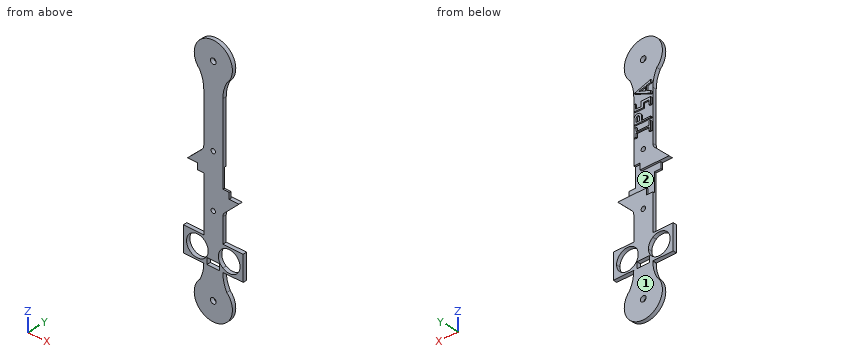
from build123d import *
from build123d.topology import SkipClean

# Parameters (mm, degrees)
SKETCH1_R            = 2
SKETCH1_R_2          = 1.5
BOSS_EXTRUDE2_DEPTH  = 3
SKETCH3_W            = 15.09800494
SKETCH3_H            = 15
CUT_EXTRUDE9_DEPTH   = 1.5
BOSS_EXTRUDE7_DEPTH  = 1.5
BOSS_EXTRUDE9_DEPTH  = 3
SKETCH11_W           = 5
SKETCH11_H           = 5
CUT_EXTRUDE16_DEPTH  = 1.5
SKETCH12_W           = 5
SKETCH12_H           = 5
BOSS_EXTRUDE16_DEPTH = 1.5
BOSS_EXTRUDE17_START = -3
SKETCH15_R           = 1.5
BOSS_EXTRUDE17_DEPTH = 3
SKETCH16_R           = 1.5
CUT_EXTRUDE17_DEPTH  = 103.05738215
BOSS_EXTRUDE23_DEPTH = 1
BOSS_EXTRUDE27_DEPTH = 3
SKETCH27_W           = 5
SKETCH27_H           = 5
CUT_EXTRUDE20_DEPTH  = 3
SKETCH28_R           = 2.25
CUT_EXTRUDE22_DEPTH  = 103.779175528
SKETCH29_R           = 1.75
CUT_EXTRUDE23_DEPTH  = 10


with BuildPart() as part:
    # Sketch1 → Boss-Extrude2 (new body)
    with BuildSketch(Plane(origin=(0, 0, 0), x_dir=(1, 0, 0), z_dir=(0, 1, 0))):
        with BuildLine():
            Line((-7.45099753, -61.780902979), (-7.45099753, 61.780902979))
            ThreePointArc((-7.45099753, 61.780902979), (-8.239083338, 68.275631842), (-10.557599248, 74.393398282))
            ThreePointArc((-10.557599248, 74.393398282), (0.04900247, 100), (10.655604188, 74.393398282))
            ThreePointArc((10.655604188, 74.393398282), (8.337088278, 68.275631842), (7.54900247, 61.780902979))
            Line((7.54900247, 61.780902979), (7.54900247, -61.780902979))
            ThreePointArc((7.54900247, -61.780902979), (8.337088278, -68.275631842), (10.655604188, -74.393398282))
            ThreePointArc((10.655604188, -74.393398282), (0.04900247, -100), (-10.557599248, -74.393398282))
            ThreePointArc((-10.557599248, -74.393398282), (-8.239083338, -68.275631842), (-7.45099753, -61.780902979))
        make_face()
        with Locations(Location((0.04900247, 85, 0), (0, 0, 270))):
            Circle(SKETCH1_R, mode=Mode.SUBTRACT)
        with Locations(Location((0, 20, 0), (0, 0, 270))):
            Circle(SKETCH1_R_2, mode=Mode.SUBTRACT)
        with Locations(Location((0.04900247, -85, 0), (0, 0, 90))):
            Circle(SKETCH1_R, mode=Mode.SUBTRACT)
        with Locations(Location((0, -20, 0), (0, 0, 90))):
            Circle(SKETCH1_R_2, mode=Mode.SUBTRACT)
    extrude(amount=BOSS_EXTRUDE2_DEPTH)

    # Sketch3 → Cut-Extrude9 (cut)
    with BuildSketch(Plane(origin=(0, 3, 0), x_dir=(1, 0, 0), z_dir=(0, 1, 0))):
        Rectangle(SKETCH3_W, SKETCH3_H)
    extrude(amount=-CUT_EXTRUDE9_DEPTH, mode=Mode.SUBTRACT)

    # Sketch4 → Boss-Extrude7 (add, symmetric)
    with BuildSketch(Plane(origin=(0, 1.5, 0), x_dir=(1, 0, 0), z_dir=(0, 1, 0))):
        Polygon((-7.380219176, -20), (-20.167033775, -7.5), (-7.45099753, -7.5), align=None)
        Polygon((7.54900247, 20), (20.167033775, 7.5), (7.54900247, 7.5), align=None)
    extrude(amount=BOSS_EXTRUDE7_DEPTH, both=True)

    # Sketch7 → Boss-Extrude9 (add)
    with BuildSketch(Plane(origin=(0, 3, 0), x_dir=(1, 0, 0), z_dir=(0, 1, 0))):
        with BuildLine():
            Line((-7.45099753, -19.930809239), (-8.881159755, -18.532726263))
            ThreePointArc((-8.881159755, -18.532726263), (-7.823107204, -20.087420247), (-7.45099753, -21.930809239))
            Line((-7.45099753, -21.930809239), (-7.45099753, -19.930809239))
        make_face()
        with BuildLine():
            Line((7.54900247, 20), (7.54900247, 22))
            ThreePointArc((7.54900247, 22), (7.918440774, 20.154044275), (8.969845829, 18.592447462))
            Line((8.969845829, 18.592447462), (7.54900247, 20))
        make_face()
    extrude(amount=-BOSS_EXTRUDE9_DEPTH)

    # Sketch11 → Cut-Extrude16 (cut)
    with BuildSketch(Plane(origin=(0, 3, 0), x_dir=(1, 0, 0), z_dir=(0, 1, 0))):
        with Locations((-4.95099753, 10)):
            Rectangle(SKETCH11_W, SKETCH11_H)
        with Locations((5.04900247, -10)):
            Rectangle(SKETCH11_W, SKETCH11_H)
    extrude(amount=-CUT_EXTRUDE16_DEPTH, mode=Mode.SUBTRACT)

    # Sketch12 → Boss-Extrude16 (add)
    with BuildSketch(Plane(origin=(0, 1.5, 0), x_dir=(1, 0, 0), z_dir=(0, 1, 0))):
        with Locations((-9.95099753, -5)):
            Rectangle(SKETCH12_W, SKETCH12_H)
        with Locations((10.04900247, 5)):
            Rectangle(SKETCH12_W, SKETCH12_H)
    extrude(amount=-BOSS_EXTRUDE16_DEPTH)

    # Sketch15 → Boss-Extrude17 (add)
    with BuildSketch(Plane(origin=(0, 3, 0), x_dir=(1, 0, 0), z_dir=(0, 1, 0)).offset(BOSS_EXTRUDE17_START)):
        with Locations((0, -20)):
            Circle(SKETCH15_R)
        with Locations((0, 20)):
            Circle(SKETCH15_R)
    extrude(amount=BOSS_EXTRUDE17_DEPTH)

    # Sketch16 → Cut-Extrude17 (cut, through all)
    with BuildSketch(Plane(origin=(0, 3, 0), x_dir=(1, 0, 0), z_dir=(0, 1, 0))):
        with Locations(Location((0, -21.2132, 0), (0, 0, 270))):
            Circle(SKETCH16_R)
        with Locations(Location((0, 21.2132, 0), (0, 0, 270))):
            Circle(SKETCH16_R)
    extrude(amount=-CUT_EXTRUDE17_DEPTH, mode=Mode.SUBTRACT)

    # Sketch23 → Boss-Extrude23 (add)
    # profile 1 of 4: a face of its own
    with BuildSketch(Plane(origin=(0, 3, 0), x_dir=(1, 0, 0), z_dir=(0, 1, 0))):
        Polygon((6.48304168, -31.15626819), (4.790546757, -31.15626819), (4.790546757, -34.224668666), (-5.193247077, -34.224668666), (-5.193247077, -31.15626819), (-6.610245289, -31.15626819), (-6.610245289, -38.224668666), (-5.172046476, -38.224668666), (-5.172046476, -35.224668666), (4.790546757, -35.224668666), (4.790546757, -38.224668666), (6.48304168, -38.224668666), align=None)
    # profile 2 of 4: a face of its own
    with BuildSketch(Plane(origin=(0, 3, 0), x_dir=(1, 0, 0), z_dir=(0, 1, 0))):
        with BuildLine():
            Line((6.48304168, -44.774262485), (6.48304168, -40.2287097))
            Line((6.48304168, -40.2287097), (0.613982134, -40.2287097))
            Line((0.613982134, -40.2287097), (-6.610245289, -40.2287097))
            Line((-6.610245289, -40.2287097), (-6.610245289, -41.2287097))
            Line((-6.610245289, -41.2287097), (0.613982134, -41.2287097))
            Line((0.613982134, -41.2287097), (0.613982134, -44.472302349))
            ThreePointArc((0.613982134, -44.472302349), (3.405099993, -47.410713479), (6.48304168, -44.774262485))
        make_face()
        with BuildLine():
            Line((2.048928068, -41.75590566), (4.790546757, -41.75590566))
            Line((4.790546757, -41.75590566), (4.790546757, -44.472302349))
            ThreePointArc((4.790546757, -44.472302349), (3.419737413, -45.843111694), (2.048928068, -44.472302349))
            Line((2.048928068, -44.472302349), (2.048928068, -41.75590566))
        make_face(mode=Mode.SUBTRACT)
    # profile 3 of 4: a face of its own
    with BuildSketch(Plane(origin=(0, 3, 0), x_dir=(1, 0, 0), z_dir=(0, 1, 0))):
        Polygon((-5.193247077, -49.786953251), (-6.610245289, -49.786953251), (-6.610245289, -55.010121906), (0.867065228, -55.010121906), (0.867065228, -51.209269606), (5.304000993, -51.209269606), (5.304000993, -55.010121906), (6.48304168, -55.010121906), (6.48304168, -54.185588488), (6.48304168, -49.786953251), (5.304000993, -49.786953251), (3.675053454, -49.786953251), (-0.919010014, -49.786953251), (-0.919010014, -53.357760144), (-5.193247077, -53.357760144), align=None)
    # profile 4 of 4: a face of its own
    with BuildSketch(Plane(origin=(0, 3, 0), x_dir=(1, 0, 0), z_dir=(0, 1, 0))):
        Polygon((6.48304168, -62.784084555), (-6.610245289, -57.417876571), (-6.610245289, -59.417876571), (-3.495842422, -60.542428347), (-3.495842422, -64.392173355), (-6.610245289, -65.17688806), (-6.610245289, -67.17688806), align=None)
        Polygon((-2.542129921, -64.151872965), (-2.542129921, -60.886795833), (2.783876522, -62.809915692), align=None, mode=Mode.SUBTRACT)
    extrude(amount=BOSS_EXTRUDE23_DEPTH)

    # Sketch18 → Boss-Extrude27 (add)
    with BuildSketch(Plane(origin=(0, 3, 0), x_dir=(1, 0, 0), z_dir=(0, 1, 0))):
        with BuildLine():
            Line((7.54900247, 44.648778007), (7.54900247, 41.473572639))
            Line((7.54900247, 41.473572639), (22.562436554, 41.473572639))
            Line((22.562436554, 41.473572639), (23.549074765, 41.473572639))
            Line((23.549074765, 41.473572639), (23.549074765, 51.473572639))
            Line((23.549074765, 51.473572639), (23.549074765, 61.473572639))
            Line((23.549074765, 61.473572639), (22.562436554, 61.473572639))
            Line((22.562436554, 61.473572639), (7.54900247, 61.473572639))
            Line((7.54900247, 61.473572639), (7.54900247, 58.424486687))
            ThreePointArc((7.54900247, 58.424486687), (16.397137863, 59.105847196), (21.029711515, 51.536632347))
            ThreePointArc((21.029711515, 51.536632347), (16.397137863, 43.967417497), (7.54900247, 44.648778007))
        make_face()
        with BuildLine():
            Line((-22.437563446, 41.473572639), (-7.45099753, 41.473572639))
            Line((-7.45099753, 41.473572639), (-7.45099753, 44.676843358))
            ThreePointArc((-7.45099753, 44.676843358), (-20.970289814, 51.536632347), (-7.45099753, 58.396421335))
            Line((-7.45099753, 58.396421335), (-7.45099753, 61.473572639))
            Line((-7.45099753, 61.473572639), (-22.437563446, 61.473572639))
            Line((-22.437563446, 61.473572639), (-23.450925235, 61.473572639))
            Line((-23.450925235, 61.473572639), (-23.450925235, 41.473572639))
            Line((-23.450925235, 41.473572639), (-22.437563446, 41.473572639))
        make_face()
    extrude(amount=-BOSS_EXTRUDE27_DEPTH)

    # Sketch27 → Cut-Extrude20 (cut)
    with SkipClean():  # the faces are left unmerged after this step: merging them gives an invalid solid
        with BuildSketch(Plane(origin=(0, 3, 0), x_dir=(1, 0, 0), z_dir=(0, 1, 0))):
            with BuildLine():
                ThreePointArc((7.54900247, 44.648778007), (16.397137863, 43.967417497), (21.029711515, 51.536632347))
                ThreePointArc((21.029711515, 51.536632347), (16.397137863, 59.105847196), (7.54900247, 58.424486687))
                Line((7.54900247, 58.424486687), (7.54900247, 44.648778007))
            make_face()
            with BuildLine():
                Line((7.54900247, 44.648778007), (7.54900247, 58.424486687))
                ThreePointArc((7.54900247, 58.424486687), (4.029711515, 51.536632347), (7.54900247, 44.648778007))
            make_face()
            with BuildLine():
                ThreePointArc((-7.45099753, 44.676843358), (-4.890250751, 47.690464411), (-3.970289814, 51.536632347))
                ThreePointArc((-3.970289814, 51.536632347), (-4.890250751, 55.382800283), (-7.45099753, 58.396421335))
                Line((-7.45099753, 58.396421335), (-7.45099753, 44.676843358))
            make_face()
            with BuildLine():
                Line((-7.45099753, 44.676843358), (-7.45099753, 58.396421335))
                ThreePointArc((-7.45099753, 58.396421335), (-20.970289814, 51.536632347), (-7.45099753, 44.676843358))
            make_face()
            with Locations((2.54900247, 58.973572639)):
                Rectangle(SKETCH27_W, SKETCH27_H)
            with Locations((-2.45099753, 58.973572639)):
                Rectangle(SKETCH27_W, SKETCH27_H)
        extrude(amount=-CUT_EXTRUDE20_DEPTH, mode=Mode.SUBTRACT)

    # Sketch28 → Cut-Extrude22 (cut, through all)
    with SkipClean():  # the faces are left unmerged after this step: merging them gives an invalid solid
        with BuildSketch(Plane(origin=(0, 3, 0), x_dir=(1, 0, 0), z_dir=(0, 1, 0))):
            with Locations(Location((0.04900247, 85, 0), (0, 0, 270))):
                Circle(SKETCH28_R)
            with Locations(Location((0.04900247, -85, 0), (0, 0, 270))):
                Circle(SKETCH28_R)
        extrude(amount=-CUT_EXTRUDE22_DEPTH, mode=Mode.SUBTRACT)

    # Sketch29 → Cut-Extrude23 (cut)
    with SkipClean():  # the faces are left unmerged after this step: merging them gives an invalid solid
        with BuildSketch(Plane(origin=(0, 3, 0), x_dir=(1, 0, 0), z_dir=(0, 1, 0))):
            with Locations(Location((0, 21.2132, 0), (0, 0, 270))):
                Circle(SKETCH29_R)
            with Locations(Location((0, -21.2132, 0), (0, 0, 270))):
                Circle(SKETCH29_R)
        extrude(amount=-CUT_EXTRUDE23_DEPTH, mode=Mode.SUBTRACT)


solid = part.part
Here's how the part is built. I have some questions about the finished solid (model axes, mm). Face numbers are marked on the shaded views. Give positions to 0.01 mm unless a question says otherwise; leave off trailing zeros. Order: outer loops, then holes, each group sorted by start corner. A loop starts at its lowest first (then second) coordinate and runs counter-clockwise, first axis right, second up. Notation, with made-up numbers: (33.5, 56) -> (74.5, 56) arc R22 cw to (74.5, 80) -> close; hole circle Ø1 at (21.25, 12.5). An arc over 180 degrees is marked (long way). Use a Markdown table: item, result. Add a question column.
Item 1: Will these pins go through, and if not, where does the flat tip stop? pin 1 (1 mm diameter, centred on x = 1, z = 62.5, fed in from +Y); pin 2 (2 mm diameter, centred on y = 3.5, z = -17.5, fed in from +X); pin 3 (0.8 mm diameter, centred on x = -4, y = 2.5, fed in from +Z); pin 4 (1.5 mm diameter, centred on x = -12, y = 2, fed in from -Z).
Item 2: Imagine slicing it at C-C on y = 0.8. Give the number of separate pieces and of enclosed holes in the cut face, plus the area to 3 significant figures.
Item 3: Imagine slicing it at D-D on z = -15.5. Please give me the cut outline in (x, y), plus the area to 3 significant figures.
Item 4: If we mould it in two halves opening along Z, with no side actions, what happens to the marked faces 1 and 2? For each: pulls with the +Z half, pulls with the -Z half, needs draft (parallel to the pull), parting line crosses it, or undercut.
Item 5: Imagine slicing it at A-A on z = 85. Please give me the cut outline in (x, y).
Item 6: I need wall thicknesses on line 1 (Z direction, x = -15, y = 2.15); line 2 (X direction, y = 1.5, z = -85); line 3 (Z direction, x = 3, y = 3.5). Which ranges of each line are inside material? Lowest first, please.
Item 7: Imagine slicing it at B-B on z = 28. Please give me the cut outline in (x, y), plus the area to 3 significant figures.
Data:
| question | item | result |
|---|---|---|
| 1 | pin 1 | stops at y = 4 |
| 1 | pin 2 | stops at x = 10.95 |
| 1 | pin 3 | stops at z = 99.55 |
| 1 | pin 4 | stops at z = -94.87 |
| 2 | separate pieces | 1 |
| 2 | enclosed holes | 7 |
| 2 | area | 3,860 mm² |
| 3 | outline | (-7.45, 0) -> (12.09, 0) -> (12.09, 3) -> (-7.45, 3) -> close |
| 3 | area | 58.6 mm² |
| 4 | face 1 | needs draft |
| 4 | face 2 | undercut |
| 5 | outline | (-14.95, 0) -> (-2.2, 0) -> (-2.2, 3) -> (-14.95, 3) -> close; (2.3, 0) -> (15.05, 0) -> (15.05, 3) -> (2.3, 3) -> close |
| 6 | line 1 | z = -61.47 to -59.65, -43.42 to -41.47, 7.5 to 12.55 |
| 6 | line 2 | x = -14.95 to -2.2, 2.3 to 15.05 |
| 6 | line 3 | z = 34.22 to 35.22, 40.23 to 41.76, 45.78 to 47.36, 49.79 to 51.21, 61.36 to 63.95 |
| 7 | outline | (-7.45, 0) -> (7.55, 0) -> (7.55, 3) -> (-7.45, 3) -> close |
| 7 | area | 45.0 mm² |
